Autodesk Fusion 360 part; units mm, degrees
sketch "Sketch1" plane through (0, 0, 0) normal (0, 0, 1) x (1, 0, 0)
  line L0 (0, 0) -> (65, 0)
  line L1 (65, 0) -> (65, 30.2)
  line L2 (65, 30.2) -> (0, 30.2)
  line L3 (0, 30.2) -> (0, 0)
  line L4 (32.5, 30.2) -> (32.5, 0)
  line L5 (65, 15.1) -> (0, 15.1)
  circle A0 centre (3.5, 26.7) radius 1.5
  circle A1 centre (61.5, 26.7) radius 1.5
  circle A2 centre (3.5, 3.7) radius 1.5
  circle A3 centre (61.5, 3.7) radius 1.5
  line L6 (7, 6.2) -> (58, 6.2)
  line L7 (58, 6.2) -> (58, 1.2)
  line L8 (58, 1.2) -> (7, 1.2)
  line L9 (7, 1.2) -> (7, 6.2)
  dimension "d1" = 65
  dimension "d2" = 30.2
  dimension "d3" = 3
  dimension "d4" = 3.5
  dimension "d5" = 3.5
  dimension "d6" = 3
  dimension "d7" = 3.5
  dimension "d8" = 3.7
  dimension "d11" = 51
  dimension "d12" = 5
  dimension "d14" = 1.2
extrude "Extrude1" add sketch "Sketch1" along normal blind 2
extrude "Extrude2" add sketch "Sketch1" against normal blind 4 contours L4 L6 L8 L9 | L4 L6 L7 L8
For this review, take the finished solid that the model builds, in its own axes (mm). A direction names the side the tool comes from. Coordinates: 2 decimals unless noted, no trailing zeros. Loops run counter-clockwise (first coordinate to the right, second up) from the corner with the lowest first, then second, coordinate; pieces in that order, holes last. Notation, with made-up numbers: (84.25, -18) -> (104.25, -18) arc R12 ccw to (104.25, -1) -> close; hole circle Ø4 at (-1, -34.75). An arc over 180 degrees is marked (long way). Return JSON: item names as keys, results as strings. Group by question number.
(1) To check wall thickness, follow L1, parallel to Y at x = 3.5, z = 0.8; L2, parallel to X at y = 4, z = 0.7; L3, parallel to X at y = 4.5, z = 1.6. State the ranges of each line that lie inside material, in increasing order.
(2) Tool access review of faces 1 (the flat face through (33, 1.2, -2)), 2 (the flat face through (7, 4, -2)), 3 (the flat face through (58, 4, -2)), 4 (the flat face through (32, 6.2, -2)): name each direction out of +Z, -Z, +X, -X, +Y, -Y from which nothing blocks a thin tool from reaching the whole face with its end or side.
(3) Consider section B-B, the plane x = 41. Give the boundary of the cut face in (y, z).
(4) Consider section A-A, the plane y = 26.7. Give the boundary of the cut face in (x, z).
(5) For pin 1 Ø3 at (x, z) = (34.5, -2.5) entering from +Y; pin 2 Ø2 at (y, z) = (3, -3) entering from -X; pin 3 Ø4 at (x, y) = (61.5, 26.7) entering from -Z, all flat-tipped, find the tip position at first contact; note any pin that passes through.
(6) Mouldability with a two-part tool opening along Y and no side actions: class faces 5 (the flat face through (32, 0, 1)), 6 (the cylindrical face through (4.306, 25.435, 0.986)), 7 (the flat face through (33, 30.2, 1)), 8 (the cylindrical face through (62.93, 26.25, 0.99)) as pulls with the +Y half, pulls with the -Y half, needs draft (parallel to the pull), parting line crosses it, or undercut.
(7) Consider section C-C, the plane x = 3.5. Give the boundary of the cut face in (y, z).
(8) Consider section D-D, the plane y = 3.7. Give the boundary of the cut face in (x, z).
Results below:
{
 "1": {"L1": "y = 0 to 2.2, 5.2 to 25.2, 28.2 to 30.2", "L2": "x = 0 to 2.03, 4.97 to 60.03, 62.97 to 65", "L3": "x = 0 to 2.23, 4.77 to 60.23, 62.77 to 65"},
 "2": {"face 1": "-Z, +X, -X, -Y", "face 2": "-Z, -X, +Y, -Y", "face 3": "-Z, +X, +Y, -Y", "face 4": "-Z, +X, -X, +Y"},
 "3": {"outline": "(0, 0) -> (1.2, 0) -> (1.2, -4) -> (6.2, -4) -> (6.2, 0) -> (30.2, 0) -> (30.2, 2) -> (0, 2) -> close"},
 "4": {"outline": "(0, 0) -> (2, 0) -> (2, 2) -> (0, 2) -> close; (5, 0) -> (60, 0) -> (60, 2) -> (5, 2) -> close; (63, 0) -> (65, 0) -> (65, 2) -> (63, 2) -> close"},
 "5": {"pin 1": "stops at y = 6.2", "pin 2": "stops at x = 7", "pin 3": "stops at z = 0"},
 "6": {"face 5": "pulls with the -Y half", "face 6": "undercut", "face 7": "pulls with the +Y half", "face 8": "undercut"},
 "7": {"outline": "(0, 0) -> (2.2, 0) -> (2.2, 2) -> (0, 2) -> close; (5.2, 0) -> (25.2, 0) -> (25.2, 2) -> (5.2, 2) -> close; (28.2, 0) -> (30.2, 0) -> (30.2, 2) -> (28.2, 2) -> close"},
 "8": {"outline": "(0, 0) -> (2, 0) -> (2, 2) -> (0, 2) -> close; (5, 0) -> (7, 0) -> (7, -4) -> (58, -4) -> (58, 0) -> (60, 0) -> (60, 2) -> (5, 2) -> close; (63, 0) -> (65, 0) -> (65, 2) -> (63, 2) -> close"}
}
